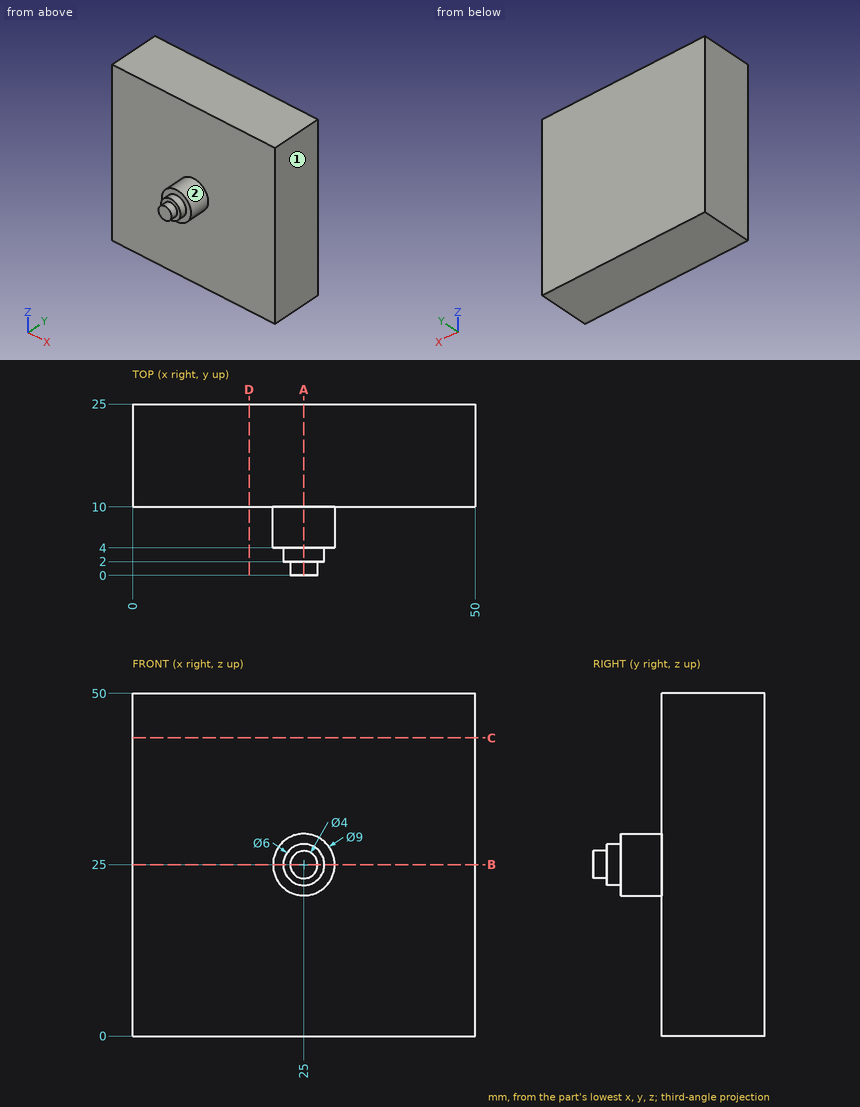
The drawing under review shows one solid part. Ordinate dimensions are in mm from its lowest x, y, z. A direction names the side the tool comes from. Coordinates: 2 decimals unless noted, no trailing zeros. Write each loop counter-clockwise with the first axis right and the second up, starting at its lowest first coordinate (ties: lowest second). Pieces come first, ordered by that corner, then holes. Notation, with made-up numbers: (66.5, 61) - (104.5, 61) arc R6 cw to (104.5, 71) - close; hole circle Ø11 at (11, 52). An arc over 180 degrees is marked (long way). Use one line per item in the form item = value.
Q1. Consider section D-D (x = 17). Write out the cut boundary in (y, z).
Taken from the geometry:
outline = (10, 0) - (25, 0) - (25, 50) - (10, 50) - close
Q2. Machinability: for the marked faces 1 and 2, which of the approach directions +Z, -Z, +X, -X, +Y, -Y give a long, thin tool a straight path to every point of the face, cutting with its end or side? Answer none if there is none.
Taken from the geometry:
face_1 = +Z, -Z, +X, +Y, -Y
face_2 = -Y
Q3. Consider section B-B (z = 25). Write out the cut boundary in (x, y), plus the area to 3 significant figures.
Taken from the geometry:
outline = (0, 10) - (20.5, 10) - (20.5, 4) - (22, 4) - (22, 2) - (23, 2) - (23, 0) - (27, 0) - (27, 2) - (28, 2) - (28, 4) - (29.5, 4) - (29.5, 10) - (50, 10) - (50, 25) - (0, 25) - close
area = 824 mm^2
Q4. Consider section A-A (x = 25). Write out the cut boundary in (y, z).
Taken from the geometry:
outline = (0, 23) - (2, 23) - (2, 22) - (4, 22) - (4, 20.5) - (10, 20.5) - (10, 0) - (25, 0) - (25, 50) - (10, 50) - (10, 29.5) - (4, 29.5) - (4, 28) - (2, 28) - (2, 27) - (0, 27) - close
Q5. Insertion check: pin 1 Ø4 at (y, z) = (7, 13) entering from -X; pin 2 Ø6 at (y, z) = (5, 24.5) entering from -X; pin 3 Ø12 at (x, z) = (30, 9.5) entering from -Y. Each pin has a flat end and moves straight along its axis. Give the tip position at first contact, or say it passes through.
Taken from the geometry:
pin_1 = through
pin_2 = 20.5
pin_3 = 10
Q6. Consider section C-C (z = 43.5). Write out the cut boundary in (x, y).
Taken from the geometry:
outline = (0, 10) - (50, 10) - (50, 25) - (0, 25) - close
Q7. For probe 1 along Y at (x, z) = (25, 14.5); probe 2 along Y at (x, z) = (23.5, 28.5), list the stretches that pass through material, from the lowest coordinate up.
Taken from the geometry:
probe_1 = 10 to 25
probe_2 = 4 to 25
